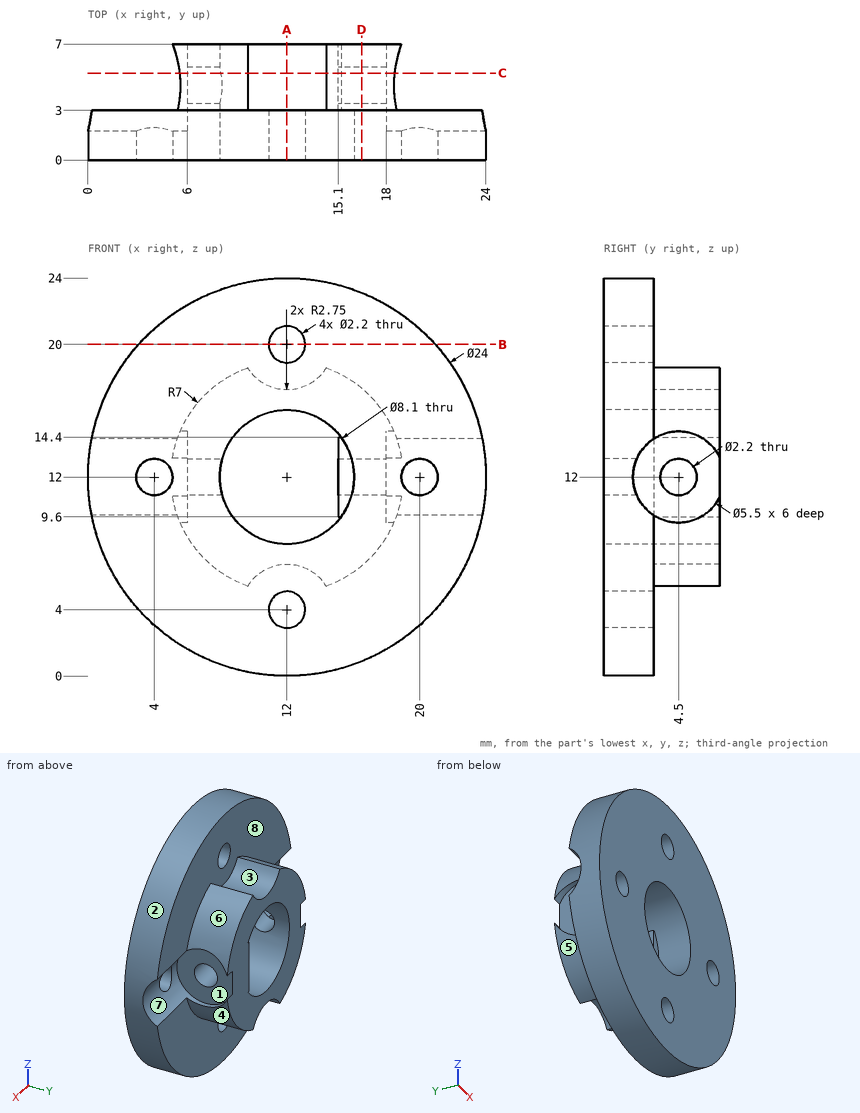
Here's the drawing with two shaded views (mm, measured from the low corner). I have some questions. A direction names the side the tool comes from. Give positions to 0.01 mm unless a question says otherwise; leave off trailing zeros. Loops run counter-clockwise (first coordinate to the right, second up) from the corner with the lowest first, then second, coordinate; pieces in that order, holes last. Notation, with made-up numbers: M 44,20 L 85,20 A23 ccw 85,46 Z; hole C 35.5,-0.5 d6. An arc over 180 degrees is marked long. One line per item, written item: value. Start each with the question number.
1) If we section it at D-D, the plane x = 16.5: Write out the boundary of the cut face in (y, z).
2) If we section it at A-A, the plane x = 12: Write out the boundary of the cut face in (y, z), and give its area (3 significant figures).
3) On a 3-axis mill with a long thin cutter (end or side, diameter ignored), from which of +Z, -Z, +X, -X, +Y, -Y can I reach the whole of each face in a straight line? I mean the marked faces 4, 5, 6, 7 and 8. Say none if no direction works.
4) If we section it at C-C, the plane y = 5.25: Write out the boundary of the cut face in (x, z), and give its area (3 significant figures).
5) If we section it at B-B, the plane z = 20: Write out the boundary of the cut face in (x, y), and give its area (3 significant figures).
6) If I drill on line 1 (X direction, y = 0.75, z = 12); line 2 (Y direction, x = 3.5, z = 20); line 3 (Z direction, x = 14, y = 0.5), over which ranges is the centre line in solid material (lowest first)? Write a range as [from, to].
7) Thinking about a two-plate mould opening in X: for the marked faces 1, 2 and 3, which applies, +X half, -X half, draft (parallel to the pull), parting line (faces both ways), or undercut?
8) I'm going to push flat-ended pins straight in: pin 1 (1.3 mm diameter, centred on x = 4, z = 12, fed in from -Y); pin 2 (5 mm diameter, centred on x = 6.5, z = 20.5, fed in from +Y); pin 3 (1 mm diameter, centred on y = 5, z = 7.5, fed in from +X); pin 4 (2.5 mm diameter, centred on y = 4, z = 11.5, fed in from -X). Where does each tip first touch, or does it pass through?
Completed:
1. outline: M 0,0.88 L 3,0.88 L 3,6.64 L 7,6.64 L 7,17.36 L 3,17.36 L 3,23.12 L 0,23.12 Z; hole C 4.5,12 d2.2
2. outline: M 0,0 L 3,0 L 3,2.9 L 0,2.9 Z; M 0,5.1 L 3,5.1 L 3,6.75 L 7,6.75 L 7,7.95 L 0,7.95 Z; M 0,16.05 L 7,16.05 L 7,17.25 L 3,17.25 L 3,18.9 L 0,18.9 Z; M 0,21.1 L 3,21.1 L 3,24 L 0,24 Z
2. area: 44.1 mm^2
3. face 4: -Z, +X, +Y
3. face 5: -Z, -X, +Y
3. face 6: +Z, +X, +Y
3. face 7: +X
3. face 8: +Z, +Y
4. outline: M 5.52,9.35 A7 ccw 9.64,5.41 A2.75 cw 14.36,5.41 A7 ccw 18.48,9.35 L 18,9.35 L 18,11.2 L 15.1,11.2 L 15.1,9.6 L 15.26,9.6 A4.05 cw 8.03,11.2 L 6,11.2 L 6,9.35 Z; M 5.52,14.65 L 6,14.65 L 6,12.8 L 8.03,12.8 A4.05 cw 15.26,14.4 L 15.1,14.4 L 15.1,12.8 L 18,12.8 L 18,14.65 L 18.48,14.65 A7 ccw 14.36,18.59 A2.75 cw 9.64,18.59 A7 ccw Z
4. area: 77.6 mm^2
5. outline: M 3.06,0 L 10.9,0 L 10.9,3 L 3.06,3 Z; M 13.1,0 L 20.94,0 L 20.94,3 L 13.1,3 Z
5. area: 47.1 mm^2
6. line 1: x = [0, 2.9], [5.1, 7.95], [16.05, 18.9], [21.1, 24]
6. line 2: y = [0, 3]
6. line 3: z = [0.17, 8.48], [15.52, 23.83]
7. face 1: +X half
7. face 2: parting line
7. face 3: undercut
8. pin 1: passes through
8. pin 2: stops at y = 3
8. pin 3: stops at x = 17.74
8. pin 4: stops at x = 6
